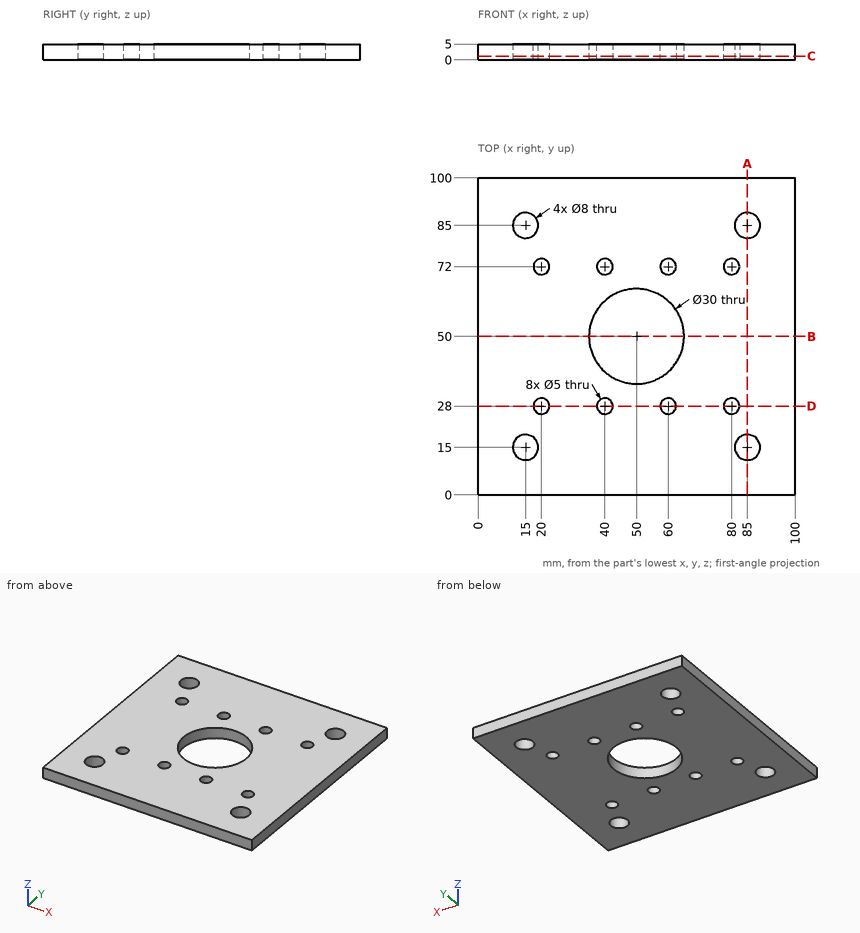
Source: three-view drawing plus pictorial views. Frame: mm from the lowest corner of the part. Round coordinates to 2 decimals unless told otherwise and drop trailing zeros. Loops run counter-clockwise (first coordinate to the right, second up) from the corner with the lowest first, then second, coordinate; pieces in that order, holes last.
Q1. Section B-B on y = 50. Return loops of the section in (x, z).
Q2. Section A-A on x = 85. Return loops of the section in (y, z).
Q3. Section C-C on z = 1.2. State how many separate pieces and enclosed holes the cut face has, plus the area to 4 significant figures.
Q4. Pin query (flat end, axial travel): P1, Ø3, axis at x = 20, y = 28, coming from the +Z side. Return the tip coordinate at first contact, or that it passes through.
Q5. Section D-D on y = 28. Return loops of the section in (x, z), plus the area to 3 significant figures.
Q6. Material intervals for L1, parallel to Y at x = 20, z = 1.05; L2, parallel to Y at x = 85, z = 2.5; L3, parallel to Y at x = 37, z = 1.7, sorted ascending.
Evaluation:
1. outline: (0, 0) - (35, 0) - (35, 5) - (0, 5) - close; (65, 0) - (100, 0) - (100, 5) - (65, 5) - close
2. outline: (0, 0) - (11, 0) - (11, 5) - (0, 5) - close; (19, 0) - (81, 0) - (81, 5) - (19, 5) - close; (89, 0) - (100, 0) - (100, 5) - (89, 5) - close
3. separate pieces: 1
3. enclosed holes: 13
3. area: 8,935 mm2
4. P1: passes through
5. outline: (0, 0) - (17.5, 0) - (17.5, 5) - (0, 5) - close; (22.5, 0) - (37.5, 0) - (37.5, 5) - (22.5, 5) - close; (42.5, 0) - (57.5, 0) - (57.5, 5) - (42.5, 5) - close; (62.5, 0) - (77.5, 0) - (77.5, 5) - (62.5, 5) - close; (82.5, 0) - (100, 0) - (100, 5) - (82.5, 5) - close
5. area: 400 mm2
6. L1: y = 0 to 25.5, 30.5 to 69.5, 74.5 to 100
6. L2: y = 0 to 11, 19 to 81, 89 to 100
6. L3: y = 0 to 42.52, 57.48 to 100
